Geometry: final body of the model. Coordinates: model frame, mm. A direction names the side the tool comes from. Give positions to 0.01 mm unless a question says otherwise; leave off trailing zeros. Loops run counter-clockwise (first coordinate to the right, second up) from the corner with the lowest first, then second, coordinate; pieces in that order, holes last. Notation, with made-up numbers: M -25.5,38 L 30.5,38 A22 ccw 30.5,49 Z; hole C 71,-11 d5. An arc over 180 degrees is marked long. Put each result on its own line as item: value.
```python
from build123d import *

# Parameters (mm, degrees)
BOSS_EXTRUDE1_DEPTH     = 5
CUT_EXTRUDE1_REACH      = 40.487
SKETCH2_W               = 51
SKETCH2_H               = 2.5
M3_5X0_6_TAPPED_HOLE4_D = 2.9
CUT_EXTRUDE2_REACH      = 40.487
CUT_EXTRUDE4_REACH      = 40.487


with BuildPart() as part:
    # Sketch1 → Boss-Extrude1 (new body)
    with BuildSketch(Plane.XY):
        Polygon((0, 0), (32.5, 0), (32.5, 20), (-32.5, 20), (-32.5, 0), align=None)
    extrude(amount=BOSS_EXTRUDE1_DEPTH)

    # Sketch2 → Cut-Extrude1 (cut, up to next)
    with BuildSketch(Plane.XZ, mode=Mode.PRIVATE) as cut_extrude1_sk1:
        with Locations((0, 1.25)):
            Rectangle(SKETCH2_W, SKETCH2_H)
    cut_extrude1_tool1 = extrude(cut_extrude1_sk1.sketch, amount=-CUT_EXTRUDE1_REACH, mode=Mode.PRIVATE) & part.part
    add(cut_extrude1_tool1.solids().sort_by_distance((0, 0, 1.25))[0], mode=Mode.SUBTRACT)

    # M3.5x0.6 Tapped Hole4 (through all)
    with Locations(Plane.XY.offset(5)):
        with Locations((-28.75, 10), (28.75, 10)):
            Hole(M3_5X0_6_TAPPED_HOLE4_D / 2)

    # Sketch12 → Cut-Extrude2 (cut, up to next)
    with BuildSketch(Plane.XY.offset(5), mode=Mode.PRIVATE) as cut_extrude2_sk1:
        Polygon((0, 20), (-10, 20), (-10, 15), (10, 15), (10, 20), align=None)
    cut_extrude2_tool1 = extrude(cut_extrude2_sk1.sketch, amount=-CUT_EXTRUDE2_REACH, mode=Mode.PRIVATE) & part.part
    add(cut_extrude2_tool1.solids().sort_by_distance((0, 17.5, 5))[0], mode=Mode.SUBTRACT)

    # Sketch14 → Cut-Extrude4 (cut, up to next)
    with BuildSketch(Plane.XZ, mode=Mode.PRIVATE) as cut_extrude4_sk1:
        Polygon((-25.5, 0), (-25.5, 0.7), (-32.5, 1.2), (-32.5, 0), align=None)
    cut_extrude4_tool1 = extrude(cut_extrude4_sk1.sketch, amount=-CUT_EXTRUDE4_REACH, mode=Mode.PRIVATE) & part.part
    add(cut_extrude4_tool1.solids().sort_by_distance((-29.307018, 0, 0.485965))[0], mode=Mode.SUBTRACT)


solid = part.part
```
Item 1: Mould query, pull axis Y, two halves, no side actions, for faces 1 (the cylindrical face through (27.411, 9.445, 2.465)), 2 (the flat face through (-24, 20, 3)), 3 (the flat face through (0, 10, 5)), 4 (the cylindrical face through (-27.3, 10.06, 2.88)). Classes: pulls with the +Y half, pulls with the -Y half, needs draft (parallel to the pull), parting line crosses it, or undercut.
Output values:
face 1: undercut
face 2: pulls with the +Y half
face 3: needs draft
face 4: undercut
Item 2: Section A-A on z = 3.5. Output: boundary loops of the cut face in (x, y), then the cut area to 3 significant figures.
Output values:
outline: M -32.5,0 L 32.5,0 L 32.5,20 L 10,20 L 10,15 L -10,15 L -10,20 L -32.5,20 Z; hole C -28.75,10 d2.9; hole C 28.75,10 d2.9
area: 1,190 mm²
Item 3: Set-up query: faces 5 (the flat face through (25.5, 10, 1)), 6 (the flat face through (32.5, 10, 2)), 7 (the flat face through (0, 15, 4)). Return all of +Z, -Z, +X, -X, +Y, -Y with unobstructed straight access to the full face (end or side cutting, diameter ignored); none if empty.
Output values:
face 5: -Z, +Y, -Y
face 6: +Z, -Z, +X, +Y, -Y
face 7: +Z, -Z, +Y
Item 4: Section B-B on y = 8. Output: boundary loops of the cut face in (x, z).
Output values:
outline: M -32.5,1.2 L -25.5,0.7 L -25.5,2.5 L 25.5,2.5 L 25.5,0 L 32.5,0 L 32.5,5 L -32.5,5 Z
Item 5: Section C-C on x = 28.75. Output: boundary loops of the cut face in (y, z), then the cut area to 3 significant figures.
Output values:
outline: M 0,0 L 8.55,0 L 8.55,5 L 0,5 Z; M 11.45,0 L 20,0 L 20,5 L 11.45,5 Z
area: 85.5 mm²
Item 6: Line query: probe 1 along Y at (x, z) = (28.75, 1.4); probe 2 along X at (y, z) = (8.25, 1.9); probe 3 along X at (y, z) = (8.75, 3.3). Output: solid intervals per line, ascending. Write a range as [from, to].
Output values:
probe 1: [0, 8.55], [11.45, 20]
probe 2: [-32.5, -25.5], [25.5, 32.5]
probe 3: [-32.5, -29.48], [-28.02, 28.02], [29.48, 32.5]
Item 7: Section D-D on x = -28.75. Output: boundary loops of the cut face in (y, z), then the cut area to 3 significant figures.
Output values:
outline: M 0,0.93 L 8.55,0.93 L 8.55,5 L 0,5 Z; M 11.45,0.93 L 20,0.93 L 20,5 L 11.45,5 Z
area: 69.6 mm²
Item 8: Pin query (flat end, axial travel): pin 1 Ø1.2 at (x, z) = (-4.5, 3.5) entering from +Y; pin 2 Ø4.5 at (x, y) = (28.75, 10) entering from +Z; pin 3 Ø2 at (x, y) = (4, 3) entering from -Z. Return the tip coordinate at first contact, or that it passes through.
Output values:
pin 1: y = 15
pin 2: z = 5
pin 3: z = 2.5
